Autodesk Inventor part; units mm, degrees
ref_plane "YZ Plane" through (0, 0, 0) normal (1, 0, 0) x (0, 1, 0)
ref_plane "XZ Plane" through (0, 0, 0) normal (0, 1, 0) x (-1, 0, 0)
ref_plane "XY Plane" through (0, 0, 0) normal (0, 0, 1) x (1, 0, 0)
sketch "Sketch1" plane through (0, 0, 0) normal (0, 1, 0) x (-1, 0, 0)
  line L0 (36, -36) -> (-36, -36)
  line L1 (-36, -36) -> (-36, 36)
  line L2 (-36, 36) -> (36, 36)
  line L3 (36, 36) -> (36, -36)
  point P0 (36, 0)
  point P1 (0, 0)
  point P2 (0, -36)
  dimension "d4" = 72
  dimension "d5" = 72
extrude "Extrusion1" add sketch "Sketch1" along normal blind 10
sketch "Sketch2" plane through (0, 10, 0) normal (0, 1, 0) x (1, 0, 0)
  point P0 (0, 0)
  point P1 (-26, -16)
  dimension "d13" = 16
  dimension "d14" = 26
hole "Hole1" at (-26, 10, 16) direction (0, -1, 0) diameter 5.5 end through all counterbore diameter 9 counterbore depth 5
pattern_linear "Rectangular Pattern1" count 2 spacing 52 along (1, 0, 0) count 2 spacing 32 along (0, 0, -1) of "Hole1"
sketch "Sketch3" plane through (0, 10, 0) normal (0, 1, 0) x (1, 0, 0)
  point P0 (0, 0)
  point P1 (0, 25)
  dimension "d28" = 25
hole "Hole2" at (0, 10, -25) direction (0, -1, 0) diameter 6.3 end through all
sketch "Sketch5" plane through (0, 0, 0) normal (0, -1, 0) x (1, 0, 0)
  circle A0 centre (0, -25) radius 3.15
  line L0 (-2.8911, -20.0025) -> (2.8824, -19.9975)
  line L1 (2.8824, -19.9975) -> (5.7735, -24.995)
  line L2 (5.7735, -24.995) -> (2.8911, -29.9975)
  line L3 (2.8911, -29.9975) -> (-2.8824, -30.0025)
  line L4 (-2.8824, -30.0025) -> (-5.7735, -25.005)
  line L5 (-5.7735, -25.005) -> (-2.8911, -20.0025)
  point P0 (0, 0)
  dimension "d38" = 10
extrude "Extrusion3" cut sketch "Sketch5" against normal blind 5 contours A0 | L0 L1 L2 L3 L4 L5
pattern_circular "Circular Pattern3" count 4 over 360 about axis through (0, -10, 0) along (0, 1, 0) of "Hole2", "Extrusion3"
sketch "Sketch6" plane through (0, 10, 0) normal (0, 1, 0) x (1, 0, 0)
  circle A0 centre (0, 0) radius 15.5
  dimension "d44" = 31
extrude "Extrusion4" add sketch "Sketch6" along normal blind 4
chamfer "Chamfer1" distance 1 angle 45 1 edges at (-15.5, 14, 0)
fillet "Fillet1" radius 20 4 edges at (-36, 5, 36) (36, 5, 36) (36, 5, -36) (-36, 5, -36)
fillet "Fillet2" radius 2 16 edges at (30.1421, 10, 30.1421) (36, 10, 0) (30.1421, 10, -30.1421) (0, 10, -36) (-30.1421, 10, -30.1421) (-36, 10, 0) (-30.1421, 10, 30.1421) (0, 10, 36) (30.1421, 0, 30.1421) (36, 0, 0) (30.1421, 0, -30.1421) (0, 0, -36) (-30.1421, 0, -30.1421) (-36, 0, 0) (-30.1421, 0, 30.1421) (0, 0, 36)
properties part number "schunk_egi_quick_release_adapter_plate"
Geometry: final body of the model. Coordinates: model frame, mm. A direction names the side the tool comes from. Give positions to 0.01 mm unless a question says otherwise; leave off trailing zeros.
(1) First-contact query: P1, Ø10, axis at x = -28, z = -15.5, coming from the +Y side; P2, Ø8, axis at x = -25, z = 0, coming from the -Y side; P3, Ø5, axis at x = 0, z = -25, coming from the -Y side; P4, Ø1, axis at x = 21, y = 6.5, coming from the +Z side. Flat tips, straight axial feed; report the tip coordinate or a pass-through.
(2) Ray query, line 1 (X direction, y = 2, z = 16); line 2 (X direction, y = 7.35, z = -16); line 3 (Z direction, x = 26, y = 2.7). Return the intervals inside material, ascending.
(3) Mould query, pull axis Z, two halves, no side actions, for faces 1 (the flat face through (-4.352, 2.465, 27.461)), 2 (the flat face through (36, 5, 0)), 3 (the flat face through (0, 5, 36)). Classes: released by +Z, released by -Z, zero draft, split by the parting line, or undercut.
(4) Access query for faces 4 (the flat face through (4.308, 2.465, 27.539)), 5 (the flat face through (26, 5, 19)), 6 (the cylindrical face through (-29.986, 5.042, -30.297)). Directions: +Z, -Z, +X, -X, +Y, -Y. A direction counts if a zero-diameter tool reaches every point of the face in a straight line with its end or side. Return the directions, or none.
(5) Cut plane A-A, the plane y = 6.5. Give the number of separate pieces and of enclosed holes in the cut face, then the cut area to 3 significant figures.
Values follow:
1. P1: stops at y = 10
1. P2: stops at y = 5
1. P3: passes through
1. P4: stops at z = 35.49
2. line 1: x = -36 to -28.75, -23.25 to 23.25, 28.75 to 36
2. line 2: x = -36 to -30.5, -21.5 to 21.5, 30.5 to 36
2. line 3: z = -33.32 to -18.75, -13.25 to -5.2, 5.19 to 13.25, 18.75 to 33.32
3. face 1: undercut
3. face 2: zero draft
3. face 3: released by +Z
4. face 4: -Y
4. face 5: +Y
4. face 6: -Z, -X, +Y, -Y
5. separate pieces: 1
5. enclosed holes: 8
5. area: 4,460 mm2
